from build123d import *

# Parameters (mm, degrees)
PAD_DEPTH         = 1.5
CHAMFER_SIZE      = 4
SKETCH001_R       = 5
SKETCH001_R_2     = 3.5
POCKET_DEPTH      = 1.501
POCKET_DEPTH_BACK = -1.501


with BuildPart() as part:
    # Sketch → Pad (new body, symmetric)
    with BuildSketch(Plane.YZ):
        Polygon((-20.25, 38), (-20.25, -38), (-11.25, -38), (-11.25, -41), (-1.25, -41), (-1.25, -38), (20.25, -38), (20.25, -25), (23.25, -25), (23.25, -15), (20.25, -15), (20.25, 15), (23.25, 15), (23.25, 25), (20.25, 25), (20.25, 38), (-1.25, 38), (-1.25, 41), (-11.25, 41), (-11.25, 38), align=None)
    extrude(amount=PAD_DEPTH, both=True)

    # Chamfer
    chamfer_edges = [part.edges().sort_by_distance(p)[0] for p in [
        (0, 20.25, 38),
        (0, 20.25, -38),
    ]]
    chamfer(chamfer_edges, length=CHAMFER_SIZE)

    # Sketch001 → Pocket (cut, two sides)
    with BuildSketch(Plane.YZ) as pocket_sk:
        Circle(SKETCH001_R)
        with Locations((-10, 20)):
            Circle(SKETCH001_R_2)
        with Locations((-10, -20)):
            Circle(SKETCH001_R_2)
    extrude(amount=-POCKET_DEPTH, mode=Mode.SUBTRACT)
    extrude(pocket_sk.sketch, amount=-POCKET_DEPTH_BACK, mode=Mode.SUBTRACT)


solid = part.part
Design review of the part built by this model. Coordinates are the model's own, in mm. A direction names the side the tool comes from. Give positions to 0.01 mm unless a question says otherwise; leave off trailing zeros. Order: outer loops, then holes, each group sorted by start corner. A loop starts at its lowest first (then second) coordinate and runs counter-clockwise, first axis right, second up.
1. Add section D-D, the plane y = -2. State the section outline as (x, z) points, then the cut area to 3 significant figures.
Solution:
outline: (-1.5, -41) - (1.5, -41) - (1.5, -4.58) - (-1.5, -4.58) - close; (-1.5, 4.58) - (1.5, 4.58) - (1.5, 41) - (-1.5, 41) - close
area: 219 mm2
2. For pin 1 Ø1.5 at (x, y) = (0, 22) entering from -Z; pin 2 Ø1.5 at (x, y) = (0, -18) entering from -Z; pin 3 Ø0.9 at (x, y) = (0, 22) entering from +Z; pin 4 Ø4 at (y, z) = (-10, 20) entering from -X, all flat-tipped, find the tip position at first contact; note any pin that passes through.
Solution:
pin 1: stops at z = -25
pin 2: stops at z = -38
pin 3: stops at z = 25
pin 4: passes through
3. To check wall thickness, follow L1, parallel to Z at x = -0.8, y = -10; L2, parallel to Y at x = 0.6, z = 0; L3, parallel to Z at x = -0.85, y = -12.5. State the ranges of each line that lie inside material, in increasing order.
Solution:
L1: z = -41 to -23.5, -16.5 to 16.5, 23.5 to 41
L2: y = -20.25 to -5, 5 to 20.25
L3: z = -38 to -22.45, -17.55 to 17.55, 22.45 to 38
4. Tool access review of faces 4 (the flat face through (0, -16, 38)), 5 (the flat face through (0, 20.25, -30)), 6 (the flat face through (0, 22, 25)), 7 (the flat face through (0, -16, -38)), 8 (the flat face through (0, 20.25, 0)): name each direction out of +Z, -Z, +X, -X, +Y, -Y from which nothing blocks a thin tool from reaching the whole face with its end or side.
Solution:
face 4: +Z, +X, -X, -Y
face 5: -Z, +X, -X, +Y
face 6: +Z, +X, -X, +Y
face 7: -Z, +X, -X, -Y
face 8: +X, -X, +Y
5. Add section A-A, the plane z = -20. State the section outline as (x, y) points.
Solution:
outline: (-1.5, -20.25) - (1.5, -20.25) - (1.5, -13.5) - (-1.5, -13.5) - close; (-1.5, -6.5) - (1.5, -6.5) - (1.5, 23.25) - (-1.5, 23.25) - close
6. Add section C-C, the plane x = 0.8. State the section outline as (y, z) points, then the cut area to 3 significant figures.
Solution:
outline: (-20.25, -38) - (-11.25, -38) - (-11.25, -41) - (-1.25, -41) - (-1.25, -38) - (16.25, -38) - (20.25, -34) - (20.25, -25) - (23.25, -25) - (23.25, -15) - (20.25, -15) - (20.25, 15) - (23.25, 15) - (23.25, 25) - (20.25, 25) - (20.25, 34) - (16.25, 38) - (-1.25, 38) - (-1.25, 41) - (-11.25, 41) - (-11.25, 38) - (-20.25, 38) - close; hole circle Ø7 at (-10, -20); hole circle Ø7 at (-10, 20); hole circle Ø10 at (0, 0)
area: 3,030 mm2
7. Mouldability with a two-part tool opening along Z and no side actions: class faces 1 (the flat face through (0, 22, 15)), 2 (the flat face through (0, -11.25, -39)), 3 (the flat face through (0, 22, -25)) as +Z half, -Z half, draft (parallel to the pull), parting line (faces both ways), or undercut.
Solution:
face 1: undercut
face 2: draft
face 3: -Z half
8. Add section B-B, the plane y = -10. State the section outline as (x, z) points, then the cut area to 3 significant figures.
Solution:
outline: (-1.5, -41) - (1.5, -41) - (1.5, -23.5) - (-1.5, -23.5) - close; (-1.5, -16.5) - (1.5, -16.5) - (1.5, 16.5) - (-1.5, 16.5) - close; (-1.5, 23.5) - (1.5, 23.5) - (1.5, 41) - (-1.5, 41) - close
area: 204 mm2
